```python
from build123d import *

# Parameters (mm, degrees)
CROQUIS1_R              = 12.5
SALIENTE_EXTRUIR1_DEPTH = 150
CROQUIS2_R              = 25
SALIENTE_EXTRUIR2_DEPTH = 7
CROQUIS3_R              = 1.5
SALIENTE_EXTRUIR3_DEPTH = 5
REDONDEO1_SIZE          = 15
REDONDEO1_SIZE_2        = 70


with BuildPart() as part:
    # Croquis1 → Saliente-Extruir1 (new body)
    with BuildSketch(Plane(origin=(0, 0, 0), x_dir=(1, 0, 0), z_dir=(0, 1, 0))):
        with Locations(Location((0, 0, 0), (0, 0, 270))):
            Circle(CROQUIS1_R)
    extrude(amount=SALIENTE_EXTRUIR1_DEPTH)

    # Croquis2 → Saliente-Extruir2 (add)
    with BuildSketch(Plane.XZ):
        with Locations(Location((0, 0, 0), (0, 0, 270))):
            Circle(CROQUIS2_R)
    extrude(amount=-SALIENTE_EXTRUIR2_DEPTH)

    # Croquis3 → Saliente-Extruir3 (add)
    with BuildSketch(Plane(origin=(0, 7, 0), x_dir=(1, 0, 0), z_dir=(0, 1, 0))):
        with BuildLine():
            Line((-7.071067812, 42.071067812), (-42.071067812, 7.071067812))
            ThreePointArc((-42.071067812, 7.071067812), (-45, 0), (-42.071067812, -7.071067812))
            Line((-42.071067812, -7.071067812), (-7.071067812, -42.071067812))
            ThreePointArc((-7.071067812, -42.071067812), (0, -45), (7.071067812, -42.071067812))
            Line((7.071067812, -42.071067812), (42.071067812, -7.071067812))
            ThreePointArc((42.071067812, -7.071067812), (45, 0), (42.071067812, 7.071067812))
            Line((42.071067812, 7.071067812), (7.071067812, 42.071067812))
            ThreePointArc((7.071067812, 42.071067812), (0, 45), (-7.071067812, 42.071067812))
        make_face()
        with Locations(Location((-35, 0, 0), (0, 0, 270))):
            Circle(CROQUIS3_R, mode=Mode.SUBTRACT)
        with Locations(Location((0, 35, 0), (0, 0, 270))):
            Circle(CROQUIS3_R, mode=Mode.SUBTRACT)
        with Locations(Location((35, 0, 0), (0, 0, 270))):
            Circle(CROQUIS3_R, mode=Mode.SUBTRACT)
        with Locations(Location((0, -35, 0), (0, 0, 270))):
            Circle(CROQUIS3_R, mode=Mode.SUBTRACT)
    extrude(amount=SALIENTE_EXTRUIR3_DEPTH)

    # Redondeo1
    # an asymmetric fillet: 70, 15 mm, written as the material it adds along each edge
    with BuildSketch(Plane(origin=(0, 12, 0), x_dir=(0, 0, 1), z_dir=(1, 0, 0))) as redondeo1_piece_1:
        with BuildLine():
            Bezier((12.5 + REDONDEO1_SIZE, REDONDEO1_SIZE * 9.99999999998e-06), (12.49985, 0.00015), (12.5 - REDONDEO1_SIZE_2 * 2.14285714285e-06, -REDONDEO1_SIZE_2), weights=[1, 0.707106781, 1])
            Line((12.5 - REDONDEO1_SIZE_2 * 2.14285714285e-06, -REDONDEO1_SIZE_2), (11.09985, -70))
            ThreePointArc((11.09985, -70), (11.1, -35), (11.1, 0))
            Line((11.1, 0), (12.5, 1.4))
            ThreePointArc((12.5, 1.4), (20, 1.4), (27.5, 1.40015))
            Line((27.5, 1.40015), (12.5 + REDONDEO1_SIZE, REDONDEO1_SIZE * 9.99999999998e-06))
        make_face()
    revolve(axis=Axis((0, 12, 0), (0, -1, 0)))


solid = part.part
```
Work out the finished part from the listing and answer in its coordinate system (mm). A direction names the side the tool comes from. Give positions to 0.01 mm unless a question says otherwise; leave off trailing zeros. Loops run counter-clockwise (first coordinate to the right, second up) from the corner with the lowest first, then second, coordinate; pieces in that order, holes last. Notation, with made-up numbers: M 74.5,21 L 85.5,21 A14 cw 85.5,32 Z; hole C 84.5,73.25 d2. An arc over 180 degrees is marked long. One line per item, written item: value. Start each with the question number.
1. Find section A-A (y = 109). Give the vertices of the cut face in (x, z).
2. Which of the six approach directions +Z, -Z, +X, -X, +Y, -Y give full straight-line access (tool end or side, diameter ignored) to faces 4 (the face through (-17, 7, 20)), 5 (the face through (3.755, 115.365, 11.923)), 6 (the face through (-0.9, 9.5, -36.2))?
3. Find the intervals of material crossed by probe 1 along Y at (x, z) = (-35.5, -8.5); probe 2 along X at (y, z) = (8.6, 35); probe 3 along Z at (x, y) = (-8.5, 101), in increasing order.
4. Find section B-B (x = 39.5). Give the vertices of the cut face in (y, z).
5. Determine the mould class of faces 1 (the face through (-0.9, 9.5, 33.8)), 2 (the face through (-27, 12, -7)), 3 (the face through (7.509, 3.451, -23.846)) for opening direction Z: released by +Z, released by -Z, zero draft, split by the parting line, or undercut.
6. Each of these flat-tipped pins is pushed along its axis until it touches: P1, Ø2.5, axis at x = 35, z = 0, coming from the +Y side; P2, Ø6, axis at y = 133.5, z = 0.5, coming from the -X side; P3, Ø1, axis at x = 0, z = -32, coming from the -Y side; P4, Ø8, axis at x = 2, y = 125, coming from the +Z side. Where does it stop, or does it pass through?
Reported:
1. outline: C 0,0 d25
2. face 4: -Y
2. face 5: +Y
2. face 6: +Y, -Y
3. probe 1: y = 7 to 12
3. probe 2: x = -14.14 to -1.5, 1.5 to 14.14
3. probe 3: z = -9.17 to 9.17
4. outline: M 7,-9.64 L 12,-9.64 L 12,9.64 L 7,9.64 Z
5. face 1: undercut
5. face 2: zero draft
5. face 3: split by the parting line
6. P1: passes through
6. P2: stops at x = -12.5
6. P3: stops at y = 7
6. P4: stops at z = 12.5
